```python
from build123d import *

# Parameters (mm, degrees)
EXTRUDE_1_DEPTH          = 1.5
CUT_EXTRUDE_1_DEPTH      = 179.051256665
CUT_EXTRUDE_1_DEPTH_BACK = 179.051256665
SKETCH_3_R               = 1.6
CUT_EXTRUDE_2_DEPTH      = 179.051256665
CUT_EXTRUDE_2_DEPTH_BACK = 179.051256665
SKETCH_4_W               = 70
SKETCH_4_H               = 15
SKETCH_4_W_2             = 30
SKETCH_4_H_2             = 5
SKETCH_5_R               = 1.6
CUT_EXTRUDE_4_DEPTH      = 179.070210872
FILLET_1_R               = 2
SKETCH_7_R               = 2.1
CUT_EXTRUDE_5_DEPTH      = 179.070210872
SKETCH_8_W               = 28
SKETCH_8_H               = 65
CUT_EXTRUDE_6_DEPTH      = 179.070210872
SKETCH_9_R               = 2.1
CUT_EXTRUDE_7_DEPTH      = 179.070210872
SKETCH_10_R              = 2.1
CUT_EXTRUDE_8_DEPTH      = 10
SKETCH_11_R              = 1.55
CUT_EXTRUDE_9_DEPTH      = 179.070210872
SKETCH_12_W              = 220
SKETCH_12_H              = 75
EXTRUDE_2_DEPTH          = 3
SKETCH_13_R              = 2.1
CUT_EXTRUDE_10_DEPTH     = 242.524325897


with BuildPart() as part:
    # 草图1 → 凸台-拉伸1 (new, symmetric)
    with BuildSketch(Plane(origin=(0, 0, 0), x_dir=(1, 0, 0), z_dir=(0, 1, 0))):
        with BuildLine():
            Line((-110, 0), (-110, 140))
            Line((-110, 140), (110, 140))
            Line((110, 140), (110, 0))
            ThreePointArc((110, 0), (0, -110), (-110, 0))
        make_face()
    extrude(amount=EXTRUDE_1_DEPTH, both=True)

    # 草图3 → 切除-拉伸1 (cut, two sides: drawn at the far end of the back side and taken through both)
    with BuildSketch(Plane(origin=(0, 0, 0), x_dir=(1, 0, 0), z_dir=(0, 1, 0)).offset(-CUT_EXTRUDE_1_DEPTH_BACK)):
        with Locations(Location((65, 90, 0), (0, 0, 270))):
            Circle(SKETCH_3_R)
        with Locations(Location((89, 90, 0), (0, 0, 270))):
            Circle(SKETCH_3_R)
        with Locations(Location((89, 60, 0), (0, 0, 270))):
            Circle(SKETCH_3_R)
        with Locations(Location((65, 60, 0), (0, 0, 270))):
            Circle(SKETCH_3_R)
        with Locations(Location((-65, 60, 0), (0, 0, 90))):
            Circle(SKETCH_3_R)
        with Locations(Location((-89, 60, 0), (0, 0, 90))):
            Circle(SKETCH_3_R)
        with Locations(Location((-89, 90, 0), (0, 0, 90))):
            Circle(SKETCH_3_R)
        with Locations(Location((-65, 90, 0), (0, 0, 90))):
            Circle(SKETCH_3_R)
    extrude(amount=CUT_EXTRUDE_1_DEPTH + CUT_EXTRUDE_1_DEPTH_BACK, mode=Mode.SUBTRACT)

    # 草图4 → 切除-拉伸2 (cut, two sides: drawn at the far end of the back side and taken through both)
    with BuildSketch(Plane(origin=(0, 0, 0), x_dir=(1, 0, 0), z_dir=(0, 1, 0)).offset(-CUT_EXTRUDE_2_DEPTH_BACK)):
        with Locations((0, 37.5)):
            Rectangle(SKETCH_4_W, SKETCH_4_H)
        with Locations((0, 116)):
            Rectangle(SKETCH_4_W_2, SKETCH_4_H_2)
    extrude(amount=CUT_EXTRUDE_2_DEPTH + CUT_EXTRUDE_2_DEPTH_BACK, mode=Mode.SUBTRACT)

    # 草图5 → 切除-拉伸4 (cut, through all)
    with BuildSketch(Plane(origin=(0, 1.5, 0), x_dir=(1, 0, 0), z_dir=(0, 1, 0))):
        with Locations(Location((-55, -30, 0), (0, 0, 270))):
            Circle(SKETCH_5_R)
        with Locations(Location((-11, -30, 0), (0, 0, 270))):
            Circle(SKETCH_5_R)
        with Locations(Location((-11, 14, 0), (0, 0, 270))):
            Circle(SKETCH_5_R)
        with Locations(Location((-55, 14, 0), (0, 0, 270))):
            Circle(SKETCH_5_R)
    extrude(amount=-CUT_EXTRUDE_4_DEPTH, mode=Mode.SUBTRACT)

    # 圆角1
    fillet_1_edges = [part.edges().sort_by_distance(p)[0] for p in [
        (35, 0, -30),
        (35, 0, -45),
        (-35, 0, -45),
        (-35, 0, -30),
    ]]
    fillet(fillet_1_edges, radius=FILLET_1_R)

    # 草图7 → 切除-拉伸5 (cut, through all)
    with BuildSketch(Plane(origin=(0, 1.5, 0), x_dir=(1, 0, 0), z_dir=(0, 1, 0))):
        with Locations(Location((-15, -60, 0), (0, 0, 270))):
            Circle(SKETCH_7_R)
        with Locations(Location((15, -60, 0), (0, 0, 270))):
            Circle(SKETCH_7_R)
        with Locations(Location((15, -84, 0), (0, 0, 270))):
            Circle(SKETCH_7_R)
        with Locations(Location((-15, -84, 0), (0, 0, 270))):
            Circle(SKETCH_7_R)
    extrude(amount=-CUT_EXTRUDE_5_DEPTH, mode=Mode.SUBTRACT)

    # 草图8 → 切除-拉伸6 (cut, through all)
    with BuildSketch(Plane(origin=(0, 1.5, 0), x_dir=(1, 0, 0), z_dir=(0, 1, 0))):
        with Locations((-113, 75)):
            Rectangle(SKETCH_8_W, SKETCH_8_H)
        with Locations((113, 75)):
            Rectangle(SKETCH_8_W, SKETCH_8_H)
    extrude(amount=-CUT_EXTRUDE_6_DEPTH, mode=Mode.SUBTRACT)

    # 草图9 → 切除-拉伸7 (cut, through all)
    with BuildSketch(Plane(origin=(0, 1.5, 0), x_dir=(1, 0, 0), z_dir=(0, 1, 0))):
        with Locations(Location((0, -102.5, 0), (0, 0, 270))):
            Circle(SKETCH_9_R)
        with Locations(Location((-72.478445072, -72.478445072, 0), (0, 0, 270))):
            Circle(SKETCH_9_R)
        with Locations(Location((-102.5, 0, 0), (0, 0, 270))):
            Circle(SKETCH_9_R)
        with Locations(Location((102.5, 0, 0), (0, 0, 270))):
            Circle(SKETCH_9_R)
        with Locations(Location((72.478445072, -72.478445072, 0), (0, 0, 270))):
            Circle(SKETCH_9_R)
    extrude(amount=-CUT_EXTRUDE_7_DEPTH, mode=Mode.SUBTRACT)

    # 草图10 → 切除-拉伸8 (cut)
    with BuildSketch(Plane(origin=(0, 1.5, 0), x_dir=(1, 0, 0), z_dir=(0, 1, 0))):
        with Locations(Location((-100, 132, 0), (0, 0, 270))):
            Circle(SKETCH_10_R)
        with Locations(Location((100, 132, 0), (0, 0, 270))):
            Circle(SKETCH_10_R)
        with Locations(Location((0, 132, 0), (0, 0, 270))):
            Circle(SKETCH_10_R)
    extrude(amount=-CUT_EXTRUDE_8_DEPTH, mode=Mode.SUBTRACT)

    # 草图11 → 切除-拉伸9 (cut, through all)
    with BuildSketch(Plane(origin=(0, 1.5, 0), x_dir=(1, 0, 0), z_dir=(0, 1, 0))):
        with Locations(Location((40, -44, 0), (0, 0, 270))):
            Circle(SKETCH_11_R)
        with Locations(Location((77.5, -44, 0), (0, 0, 270))):
            Circle(SKETCH_11_R)
        with Locations(Location((77.5, 17.5, 0), (0, 0, 270))):
            Circle(SKETCH_11_R)
        with Locations(Location((40, 17.5, 0), (0, 0, 270))):
            Circle(SKETCH_11_R)
    extrude(amount=-CUT_EXTRUDE_9_DEPTH, mode=Mode.SUBTRACT)

    # 草图12 → 凸台-拉伸2 (add)
    with BuildSketch(Plane(origin=(0, 1.5, 0), x_dir=(1, 0, 0), z_dir=(0, 1, 0))):
        with Locations((0, 177.5)):
            Rectangle(SKETCH_12_W, SKETCH_12_H)
    extrude(amount=-EXTRUDE_2_DEPTH)

    # 草图13 → 切除-拉伸10 (cut, through all)
    with BuildSketch(Plane(origin=(0, 1.5, 0), x_dir=(1, 0, 0), z_dir=(0, 1, 0))):
        with Locations(Location((100, 209, 0), (0, 0, 270))):
            Circle(SKETCH_13_R)
        with Locations(Location((-100, 209, 0), (0, 0, 90))):
            Circle(SKETCH_13_R)
    extrude(amount=-CUT_EXTRUDE_10_DEPTH, mode=Mode.SUBTRACT)


solid = part.part
```
Check sheet for the modelled part. Datum: model origin and axes. Units: mm. Give positions to 0.01 mm unless a question says otherwise; leave off trailing zeros.
Item 1: Gauge pin test, flat end, axial feed: pin 1 (1.5 mm diameter, centred on y = -0.5, z = 23.5, fed in from -X). Record the tip position at first contact, or that the pin passes through.
Item 2: Cross-section at A-A (y = -0.05). Count the separate pieces of the cut face and the enclosed holes in it, and give its area (3 significant figures).
Item 3: Draft check along Z on faces 1 (the face through (-2, 1.5, -55)), 2 (the face through (2.419, 0.021, 109.973)). Enter one of: released by +Z, released by -Z, zero draft, split by the parting line, or undercut.
Item 4: Scan lines: L1, parallel to X at y = 0.6, z = -90; L2, parallel to X at y = -0.25, z = -132; L3, parallel to Z at x = 77, y = -0.8. Record each from-to range of solid material in increasing order.
Report:
1. pin 1: stops at x = -107.62
2. separate pieces: 1
2. enclosed holes: 32
2. area: 63,400 mm2
3. face 1: zero draft
3. face 2: released by +Z
4. L1: x = -99 to -90.6, -87.4 to -66.6, -63.4 to 63.4, 66.6 to 87.4, 90.6 to 99
4. L2: x = -110 to -102.1, -97.9 to -2.1, 2.1 to 97.9, 102.1 to 110
4. L3: z = -215 to -18.97, -16.03 to 42.53, 45.47 to 78.56
